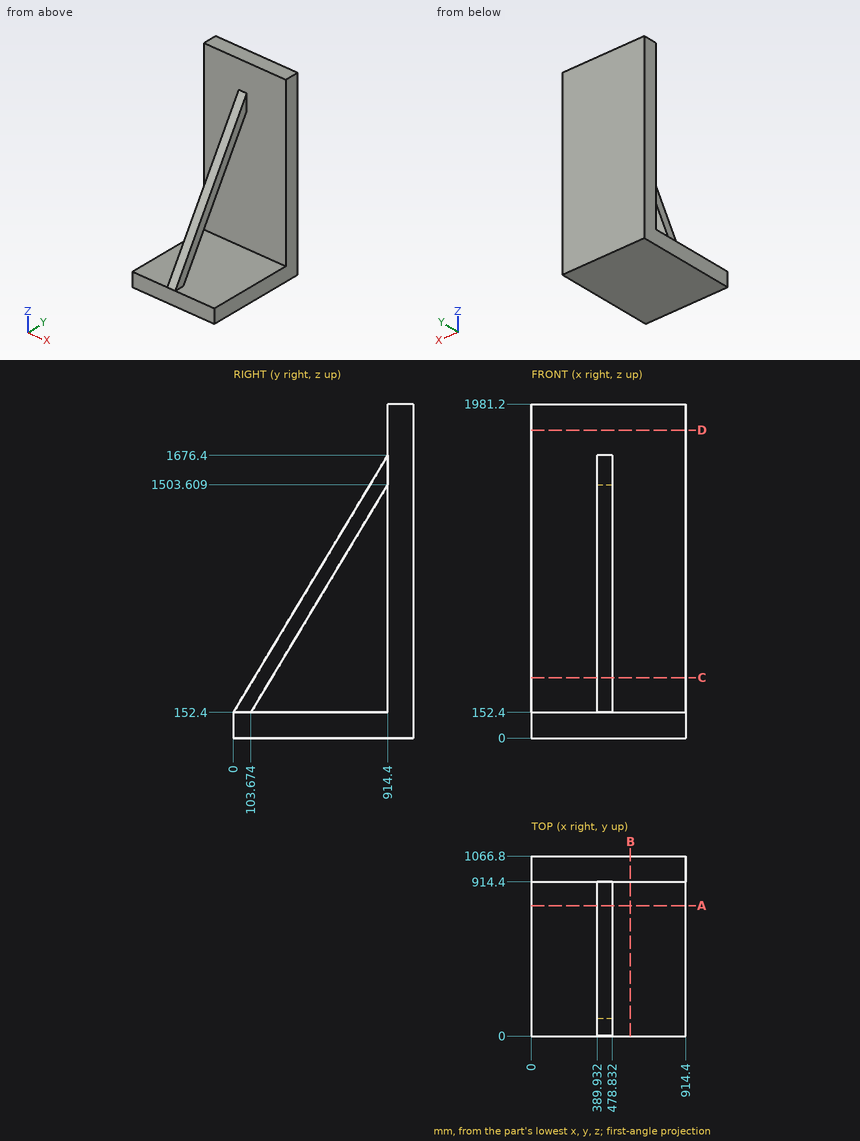
Answer from the drawing. Dimensions are ordinates in mm from the lowest x, y and z of the part. Round coordinates to 2 decimals unless told otherwise and drop trailing zeros. Write each loop counter-clockwise with the first axis right and the second up, starting at its lowest first coordinate (ties: lowest second). Pieces come first, ordered by that corner, then holes.
1. Straight lines are drawn through the part: L1, parallel to Y at x = 307, z = 238.5; L2, parallel to Z at x = 226.5, y = 648; L3, parallel to X at y = 828.5, z = 1496.5. For each, find the intervals that lie inside material, in ascending order.
2. The part is cut by section A-A, the plane y = 773. Determine the outline of the cut face in (x, z), then the cut area to 3 significant figures.
3. The part is cut by section C-C, the plane z = 358. Determine the outline of the cut face in (x, y) (1 decimal).
4. The part is cut by section D-D, the plane z = 1826. Determine the outline of the cut face in (x, y), then the cut area to 3 significant figures.
5. Given pin 1 Ø3 at (x, y) = (208, 574) entering from +Z; pin 2 Ø6 at (x, z) = (714.5, 1031.5) entering from -Y, each flat-ended and moving along its own axis, determine where each tip first touches the part or whether it passes through.
6. The part is cut by section B-B, the plane x = 586.5. Determine the outline of the cut face in (y, z), then the cut area to 3 significant figures.
Values:
1. L1: y = 914.4 to 1066.8
1. L2: z = 0 to 152.4
1. L3: x = 389.93 to 478.83
2. outline: (0, 0) - (914.4, 0) - (914.4, 152.4) - (0, 152.4) - close; (389.93, 1267.94) - (478.83, 1267.94) - (478.83, 1440.73) - (389.93, 1440.73) - close
2. area: 155,000 mm2
3. outline: (0, 914.4) - (914.4, 914.4) - (914.4, 1066.8) - (0, 1066.8) - close; (389.9, 123.4) - (478.8, 123.4) - (478.8, 227) - (389.9, 227) - close
4. outline: (0, 914.4) - (914.4, 914.4) - (914.4, 1066.8) - (0, 1066.8) - close
4. area: 139,000 mm2
5. pin 1: stops at z = 152.4
5. pin 2: stops at y = 914.4
6. outline: (0, 0) - (1066.8, 0) - (1066.8, 1981.2) - (914.4, 1981.2) - (914.4, 152.4) - (0, 152.4) - close
6. area: 441,000 mm2
